Design review of the part built by this model. Coordinates are the model's own, in mm. Face numbers are marked on the shaded views. A direction names the side the tool comes from. Give positions to 0.01 mm unless a question says otherwise; leave off trailing zeros. Order: outer loops, then holes, each group sorted by start corner. A loop starts at its lowest first (then second) coordinate and runs counter-clockwise, first axis right, second up. Notation, with made-up numbers: (29.25, 82.5) - (40.25, 82.5) arc R20 cw to (40.25, 98.5) - close; hole circle Ø1 at (-23, -34.5). An arc over 180 degrees is marked (long way). Write each question's results on one line, items separated by ' | '. Start each with the question number.
```python
from build123d import *

# Parameters (mm, degrees)
F0_W     = 20
F0_H     = 17
F0_W_2   = 17
F0_H_2   = 77
F1_DEPTH = 8.5
F3_DEPTH = 20
F4_DEPTH = 20
F5_R     = 8


with BuildPart() as f1:
    # F0 (on Front) → F1 (new body, symmetric)
    with BuildSketch(Plane.XZ):
        with Locations((-10, 8.5)):
            Rectangle(F0_W, F0_H)
        Polygon((-37, 0), (-20, 0), (-20, 17), (-28.5, 8.5), align=None)
        with Locations((-28.5, 55.5)):
            Rectangle(F0_W_2, F0_H_2)
        Polygon((-28.5, 8.5), (-20, 17), (-37, 17), align=None)
        Polygon((-37, 17), (-37, 0), (-28.5, 8.5), align=None)
        Polygon((-37, 94), (-20, 94), (-20, 111), (-28.5, 102.5), align=None)
        with Locations((-10, 102.5)):
            Rectangle(F0_W, F0_H)
        Polygon((-28.5, 102.5), (-20, 111), (-37, 111), align=None)
        Polygon((-37, 111), (-37, 94), (-28.5, 102.5), align=None)
    extrude(amount=F1_DEPTH, both=True)

    # F2 (on face) → F3 (cut)
    with BuildSketch(Plane.YZ):
        with BuildLine():
            ThreePointArc((1.75, 102.5), (0.6696960066, 104.1167891819), (-1.2374368671, 103.7374368671))
            Line((-1.2374368671, 103.7374368671), (0, 102.5))
            Line((0, 102.5), (1.2374368671, 101.2625631329))
            ThreePointArc((1.2374368671, 101.2625631329), (1.6167891819, 101.8303039934), (1.75, 102.5))
        make_face()
        with BuildLine():
            Line((1.2374368671, 101.2625631329), (0, 102.5))
            Line((0, 102.5), (-1.2374368671, 101.2625631329))
            ThreePointArc((-1.2374368671, 101.2625631329), (0, 100.75), (1.2374368671, 101.2625631329))
        make_face()
        with BuildLine():
            Line((0, 102.5), (-1.2374368671, 103.7374368671))
            ThreePointArc((-1.2374368671, 103.7374368671), (-1.75, 102.5), (-1.2374368671, 101.2625631329))
            Line((-1.2374368671, 101.2625631329), (0, 102.5))
        make_face()
    extrude(amount=-F3_DEPTH, mode=Mode.SUBTRACT)

    # F2 (on face) → F4 (cut)
    with BuildSketch(Plane.YZ):
        with BuildLine():
            Line((0, 8.5), (-1.2374368671, 7.2625631329))
            ThreePointArc((-1.2374368671, 7.2625631329), (0, 6.75), (1.2374368671, 7.2625631329))
            Line((1.2374368671, 7.2625631329), (0, 8.5))
        make_face()
        with BuildLine():
            Line((1.2374368671, 9.7374368671), (0, 8.5))
            Line((0, 8.5), (1.2374368671, 7.2625631329))
            ThreePointArc((1.2374368671, 7.2625631329), (1.6167891819, 7.8303039934), (1.75, 8.5))
            ThreePointArc((1.75, 8.5), (1.6167891819, 9.1696960066), (1.2374368671, 9.7374368671))
        make_face()
        with BuildLine():
            ThreePointArc((1.2374368671, 9.7374368671), (-1.2374368671, 9.7374368671), (-1.2374368671, 7.2625631329))
            Line((-1.2374368671, 7.2625631329), (0, 8.5))
            Line((0, 8.5), (1.2374368671, 9.7374368671))
        make_face()
    extrude(amount=-F4_DEPTH, mode=Mode.SUBTRACT)

    # F5
    f5_edges = [f1.edges().sort_by_distance(p)[0] for p in [
        (-20, 8.5, 55.5),
        (-20, -8.5, 55.5),
        (-10, 8.5, 94),
        (-10, -8.5, 94),
        (-10, -8.5, 17),
        (-10, 8.5, 17),
        (-18.5, -8.5, 0),
        (-18.5, 8.5, 0),
        (-18.5, -8.5, 111),
        (-18.5, 8.5, 111),
    ]]
    fillet(f5_edges, radius=F5_R)


solid = f1.part
```
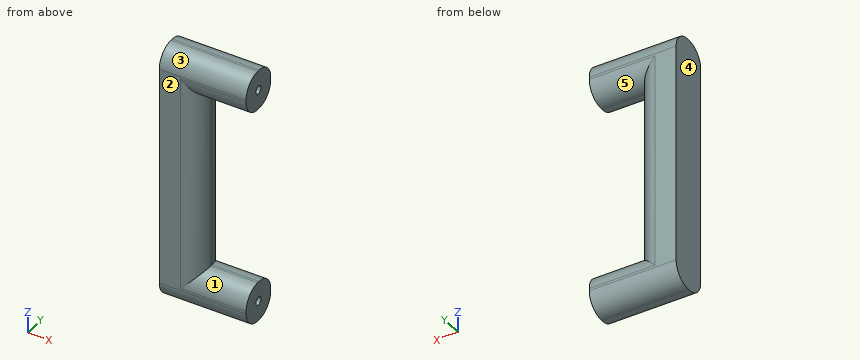
Q1. Machinability: for the marked faces 1 and 2, which of the approach directions +Z, -Z, +X, -X, +Y, -Y give a long, thin tool a straight path to every point of the face, cutting with its end or side? Answer none if there is none.
Q2. Draft analysis for pull direction Z (two halves, no side actions). For the marked faces 3, 4 and 5, state which applies: pulls with the +Z half, pulls with the -Z half, needs draft (parallel to the pull), parting line crosses it, or undercut.
Q3. Insertion check: pin 1 Ø3 at (y, z) = (0.5, 50.5) entering from +X; pin 2 Ø6 at (x, y) = (-5, -5) entering from +Z; pin 3 Ø1 at (x, y) = (-7.5, -3.5) entering from +Z. Each pin has a flat end and moves straight along its axis. Give the tip position at first contact, or say it passes through.
Q4. Add section C-C (y = 3). Give the boundary of the cut face in (x, z), plus the area to 3 significant figures.
Q5. For line 1 (Z direction, x = -10, y = 1.25); line 2 (X direction, y = 0.75, z = 51.5); line 3 (Z direction, x = -20, y = -5), list the stretches that pass through material, from the lowest coordinate up. Write a range as [from, to].
Q6. Add section A-A (x = -19). Give the boundary of the cut face in (y, z).
Q7. Add section B-B (z = 37). Give the boundary of the cut face in (x, y), plus the area to 3 significant figures.
Verdict:
1) face 1: +X, -Y | face 2: +Z, -Z, +X, -X, -Y
2) face 3: pulls with the +Z half | face 4: needs draft | face 5: undercut
3) pin 1: stops at x = -20 | pin 2: stops at z = 110.86 | pin 3: stops at z = 110.6
4) outline: (-37, 0.4) - (0, 0.4) - (0, 16.6) - (-20.4, 16.6) - (-20.4, 94.4) - (0, 94.4) - (0, 110.6) - (-37, 110.6) - close | area: 2,490 mm2
5) line 1: z = [0.04, 7.28], [9.72, 16.96], [94.04, 101.28], [103.72, 110.96] | line 2: x = [-37, -20] | line 3: z = [1.39, 15.61], [95.39, 109.61]
6) outline: (-8.5, 8) arc R8 ccw to (-0.5, 0) - (0.5, 0) arc R8 ccw to (8.5, 8) - (8.5, 9) arc R8 ccw to (0.5, 17) - (-0.5, 17) arc R8 ccw to (-8.5, 9) - close; (-8.5, 102) arc R8 ccw to (-0.5, 94) - (0.5, 94) arc R8 ccw to (8.5, 102) - (8.5, 103) arc R8 ccw to (0.5, 111) - (-0.5, 111) arc R8 ccw to (-8.5, 103) - close; hole circle Ø3.5 at (0, 8.5); hole circle Ø3.5 at (0, 102.5)
7) outline: (-37, -8.5) - (-28, -8.5) arc R8 ccw to (-20, -0.5) - (-20, 0.5) arc R8 ccw to (-28, 8.5) - (-37, 8.5) - close | area: 262 mm2
